Design review of the part shown in the three views and the two pictorial views. Dimensions are in mm from the part's minimum x, y and z. A direction names the side the tool comes from. Coordinates: 2 decimals unless noted, no trailing zeros. Loops run counter-clockwise (first coordinate to the right, second up) from the corner with the lowest first, then second, coordinate; pieces in that order, holes last. Notation, with made-up numbers: M 81,3.25 L 131,3.25 A15 ccw 131,19.25 Z; hole C 23.25,-23.5 d7. An arc over 180 degrees is marked long. Put each result on its own line as item: value. Start each with the question number.
(1) Clearance check with flat-ended pins moving along their axes: pin 1 (2.5 mm diameter, centred on y = 6.5, z = 20.5, fed in from -X); pin 2 (3 mm diameter, centred on x = 10.5, z = 10, fed in from -Y); pin 3 (8 mm diameter, centred on x = 16.5, y = 7, fed in from -Z); pin 4 (5 mm diameter, centred on y = 19.5, z = 9, fed in from -X). State where each tip first meets the part, or that it passes through.
(2) Take a section at A-A, the plane z = 21. Give the boundary of the cut face in (x, y) (1 decimal).
(3) Take a section at D-D, the plane x = 29. Give the boundary of the cut face in (y, z) (1 decimal).
(4) Take a section at B-B, the plane x = 5. Give the boundary of the cut face in (y, z) (1 decimal).
(5) For the marked faces 1, 2 and 3, list the 3-axis set-ups (+Z, -Z, +X, -X, +Y, -Y) from which the entire face can be reached by the end or side of a thin tool; tool diameter is ignored.
(6) For probe 1 along X at (y, z) = (12, 19.5); probe 2 along Z at (x, y) = (7.5, 24.25) (1 decimal); probe 3 along Z at (x, y) = (23.5, 10.5) (1 decimal), list the stretches that pass through material, from the lowest coordinate up. Write a range as [from, to].
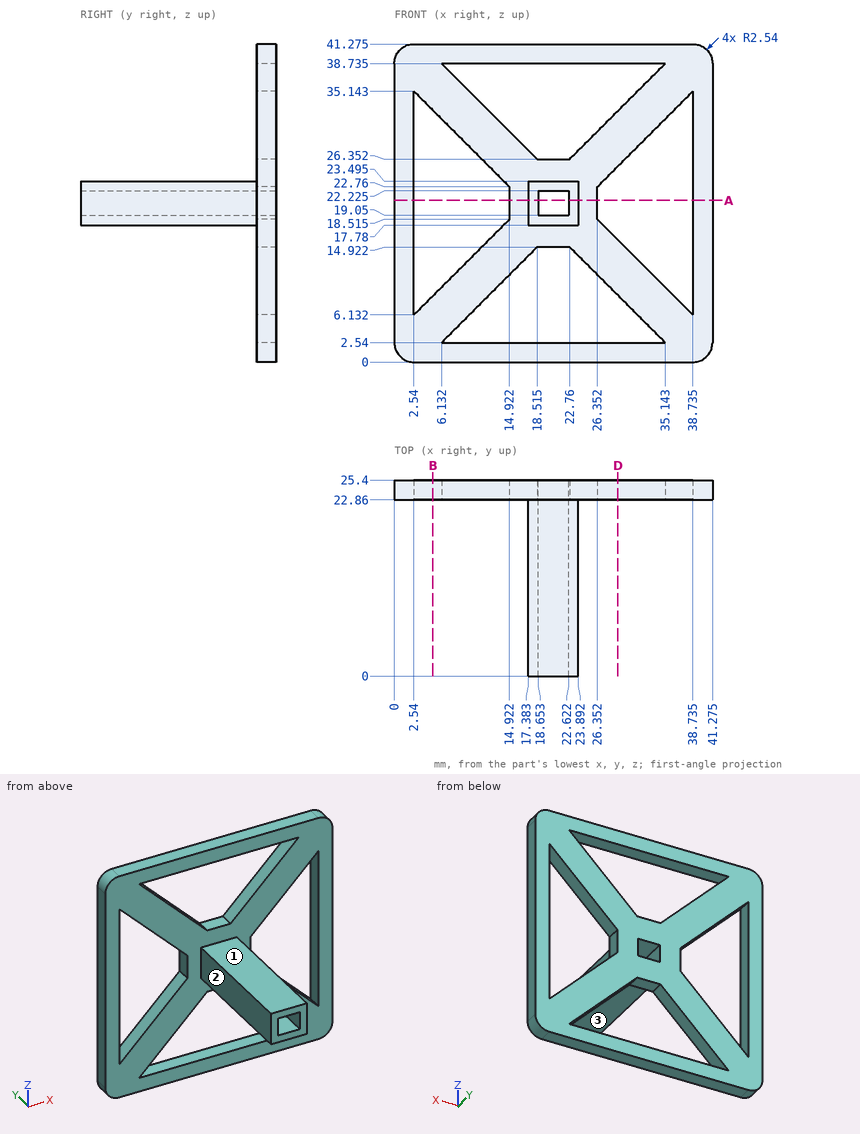
Computed values:
1. pin 1: stops at x = 17.38
1. pin 2: stops at y = 22.86
1. pin 3: stops at z = 17.78
1. pin 4: passes through
2. outline: M 0,22.9 L 2.5,22.9 L 2.5,25.4 L 0,25.4 Z; M 14.9,22.9 L 17.4,22.9 L 17.4,0 L 18.7,0 L 18.7,25.4 L 14.9,25.4 Z; M 22.6,0 L 23.9,0 L 23.9,22.9 L 26.4,22.9 L 26.4,25.4 L 22.6,25.4 Z; M 38.7,22.9 L 41.3,22.9 L 41.3,25.4 L 38.7,25.4 Z
3. outline: M 22.9,0 L 25.4,0 L 25.4,2.5 L 22.9,2.5 Z; M 22.9,8.7 L 25.4,8.7 L 25.4,15.9 L 22.9,15.9 Z; M 22.9,25.4 L 25.4,25.4 L 25.4,32.6 L 22.9,32.6 Z; M 22.9,38.7 L 25.4,38.7 L 25.4,41.3 L 22.9,41.3 Z
4. outline: M 22.9,0 L 25.4,0 L 25.4,8.6 L 22.9,8.6 Z; M 22.9,32.7 L 25.4,32.7 L 25.4,41.3 L 22.9,41.3 Z
5. face 1: +Z, +X, -X, -Y
5. face 2: +Z, -Z, -X, -Y
5. face 3: -Z, +X, -X, -Y
6. probe 1: x = [17.38, 18.65], [22.62, 23.89]
6. probe 2: z = [0, 2.5], [3.9, 11.1], [30.2, 37.4], [38.7, 41.3]
6. probe 3: z = [17.8, 23.5]
